Here's the drawing with two shaded views (mm, measured from the low corner). I have some questions. A direction names the side the tool comes from. Give positions to 0.01 mm unless a question says otherwise; leave off trailing zeros. Loops run counter-clockwise (first coordinate to the right, second up) from the corner with the lowest first, then second, coordinate; pieces in that order, holes last. Notation, with made-up numbers: (25, 43.25) - (35, 43.25) arc R14 ccw to (35, 66.25) - close; hole circle Ø7 at (62, -25.5). An arc over 180 degrees is marked (long way). Use a Markdown table: item, result. Add a question column.
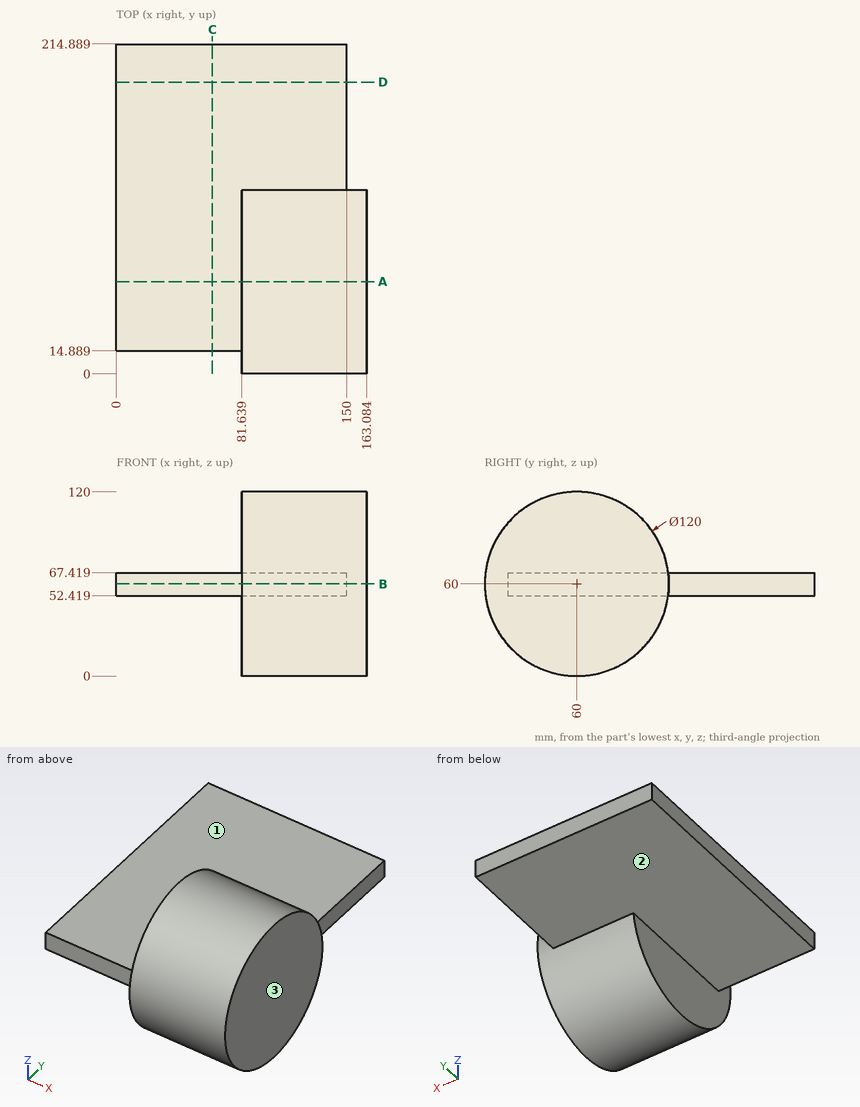
1. On a 3-axis mill with a long thin cutter (end or side, diameter ignored), from which of +Z, -Z, +X, -X, +Y, -Y can I reach the whole of each face in a straight line? I mean the marked faces 1, 2 and 3. Say none if no direction works.
2. Please list where these lines run through material, in increasing order: line 1 along X through (y, z) = (56.5, 114) (1 decimal); line 2 along Z through (x, y) = (10, 182.5); line 3 along Y through (x, z) = (103, 19.5). Write a range as [from, to].
3. Will these pins go through, and if not, where does the flat tip stop? P1, Ø4, axis at x = 117, y = 27, coming from the +Z side; P2, Ø12, axis at x = 67.5, y = 90.5, coming from the -Z side; P3, Ø7.5, axis at y = 187.5, z = 63.5, coming from the +X side.
4. Suppose I cut it at A-A (y = 60). List the corners of the cut face in (x, z) for me (1 decimal).
5. Suppose I cut it at B-B (z = 60). List the corners of the cut face in (x, y) for me (1 decimal), and give its area (3 significant figures).
6. Suppose I cut it at D-D (y = 190). List the corners of the cut face in (x, z) for me, and give its area (3 significant figures).
7. Suppose I cut it at C-C (x = 62.5). List the corners of the cut face in (y, z) for me.
Results below:
| question | item | result |
|---|---|---|
| 1 | face 1 | +Z, -X, +Y |
| 1 | face 2 | -Z, -X, +Y |
| 1 | face 3 | +Z, -Z, +X, +Y, -Y |
| 2 | line 1 | [81.6, 163.1] |
| 2 | line 2 | [52.42, 67.42] |
| 2 | line 3 | [15.73, 104.27] |
| 3 | P1 | z = 111.37 |
| 3 | P2 | z = 52.42 |
| 3 | P3 | x = 150 |
| 4 | outline | (0, 52.4) - (81.6, 52.4) - (81.6, 0) - (163.1, 0) - (163.1, 120) - (81.6, 120) - (81.6, 67.4) - (0, 67.4) - close |
| 5 | outline | (0, 14.9) - (81.6, 14.9) - (81.6, 0) - (163.1, 0) - (163.1, 120) - (150, 120) - (150, 214.9) - (0, 214.9) - close |
| 5 | area | 32,600 mm² |
| 6 | outline | (0, 52.42) - (150, 52.42) - (150, 67.42) - (0, 67.42) - close |
| 6 | area | 2,250 mm² |
| 7 | outline | (14.89, 52.42) - (214.89, 52.42) - (214.89, 67.42) - (14.89, 67.42) - close |
